Autodesk Inventor part; units mm, degrees
ref_plane "YZ Plane" through (0, 0, 0) normal (1, 0, 0) x (0, 1, 0)
ref_plane "XZ Plane" through (0, 0, 0) normal (0, 1, 0) x (-1, 0, 0)
ref_plane "XY Plane" through (0, 0, 0) normal (0, 0, 1) x (1, 0, 0)
sketch "Sketch1" plane through (0, 0, 0) normal (0, 0, 1) x (1, 0, 0)
  circle A0 centre (0, 0) radius 2.5
  line L0 (0, 0) -> (-10.5, 0)
  circle A1 centre (-10.5, 0) radius 1.5
  arc A2 (-10.5, 5) -> (-10.5, -5) centre (-10.5, 0) ccw
  line L1 (-10.5, 5) -> (0, 5)
  line L2 (0, 5) -> (0, -5)
  line L3 (0, -5) -> (-10.5, -5)
  line L4 (0, 0) -> (0, -10.5)
  circle A3 centre (0, -10.5) radius 1.5
  arc A4 (-5, -10.5) -> (5, -10.5) centre (0, -10.5) ccw
  line L5 (-5, -10.5) -> (-5, 0)
  line L6 (5, 0) -> (5, -10.5)
  line L7 (0, 0) -> (10.5, 0)
  circle A5 centre (10.5, 0) radius 1.5
  arc A6 (10.5, -5) -> (10.5, 5) centre (10.5, 0) ccw
  line L8 (10.5, -5) -> (0, -5)
  line L9 (0, 5) -> (10.5, 5)
  line L10 (0, 0) -> (0, 10.5)
  circle A7 centre (0, 10.5) radius 1.5
  arc A8 (5, 10.5) -> (-5, 10.5) centre (0, 10.5) ccw
  line L11 (5, 10.5) -> (5, 0)
  line L12 (-5, 0) -> (-5, 10.5)
  circle A9 centre (0, 0) radius 4.5
  point P0 (-5, -5)
  point P1 (5, -5)
  point P2 (5, 5)
  point P3 (-5, 5)
  dimension "d0" = 10.5
  dimension "d1" = 3
  dimension "d2" = 5
  dimension "d3" = 10
  dimension "d6" = 360
  dimension "d8" = 9
extrude "Extrusion1" add sketch "Sketch1" against normal blind 2 contours L7 A9 L2 A0 | A0 L2 A9 L7 | A0 L0 A9 L2 | L2 A9 L0 A0 | A9 L2 L9 L11 L7 | L7 L6 L8 L2 A9 | A9 L0 L12 L1 L2 | L2 L3 L5 L0 A9 | L11 L9 A6 L8 L6 | L1 L12 A8 L11 L9 | L8 L6 A4 L5 L3 | L5 L3 A2 L1 L12
extrude "Extrusion2" add sketch "Sketch1" along normal blind 10 contours L7 A9 L2 A0 | A0 L2 A9 L7 | A0 L0 A9 L2 | L2 A9 L0 A0
fillet "Fillet1" radius 1 12 edges at (-7.75, -5, 0) (-7.75, 5, 0) (-15.5, 0, 0) (5, -7.75, 0) (-5, -7.75, 0) (0, -15.5, 0) (15.5, 0, 0) (7.75, 5, 0) (7.75, -5, 0) (-5, 7.75, 0) (5, 7.75, 0) (0, 15.5, 0)
chamfer "Chamfer1" distance 1 angle 45 1 edges at (-4.5, 0, 0)
fillet "Fillet2" radius 1 1 edges at (-4.5, 0, 10)
properties part number "dudukan gps"
Input: part model. Units: mm. Frame: model coordinates. A direction names the side the tool comes from. Coordinates: 2 decimals unless noted, no trailing zeros. Order: outer loops, then holes, each group sorted by start corner. A loop starts at its lowest first (then second) coordinate and runs counter-clockwise, first axis right, second up. Notation, with made-up numbers: (39.25, 59.25) - (45.25, 59.25) arc R28 cw to (45.25, 97.25) - close; hole circle Ø7 at (88.5, 10.25). An arc over 180 degrees is marked (long way). Put each result on its own line as item: value.
1. Reachability of faces 1 (the face through (7.296, -4.699, -0.285)), 2 (the face through (-4.715, -7.204, -0.301)), 3 (the face through (4.715, 7.204, -0.301)), 4 (the face through (7.8, -5, -1.5)), 5 (the face through (-7.204, 4.715, -0.301)) from +Z, -Z, +X, -X, +Y, -Y: full face, straight path, thin tool, end or side. Return the list, or none.
Report:
face 1: +Z, +X, -Y
face 2: +Z, -X, -Y
face 3: +Z, +X, +Y
face 4: +Z, -Z, +X, -Y
face 5: +Z, -X, +Y
2. Line query: line 1 along Y through (x, z) = (0, -1.1); line 2 along X through (y, z) = (-10.5, -1.5); line 3 along X through (y, z) = (0, 1.25). Output: solid intervals per line, ascending.
Report:
line 1: y = -15.5 to -12, -9 to -2.5, 2.5 to 9, 12 to 15.5
line 2: x = -5 to -1.5, 1.5 to 5
line 3: x = -4.5 to -2.5, 2.5 to 4.5
3. Draft query along X for faces 6 (the face through (0, -12, -1)), 7 (the face through (7.7, 5, -1.5)), 8 (the face through (-15.5, 0.1, -1.5)), 9 (the face through (-12, 0, -1)). Return one class per face: pulls with the +X half, pulls with the -X half, needs draft (parallel to the pull), parting line crosses it, or undercut.
Report:
face 6: undercut
face 7: needs draft
face 8: pulls with the -X half
face 9: undercut
4. Cut plane A-A on y = 0. Return the cut outline in (x, z).
Report:
outline: (-15.5, -2) - (-12, -2) - (-12, 0) - (-14.5, 0) arc R1 ccw to (-15.5, -1) - close; (-9, -2) - (-2.5, -2) - (-2.5, 10) - (-3.5, 10) arc R1 ccw to (-4.5, 9) - (-4.5, 1) - (-5.5, 0) - (-9, 0) - close; (2.5, -2) - (9, -2) - (9, 0) - (5.5, 0) - (4.5, 1) - (4.5, 9) arc R1 ccw to (3.5, 10) - (2.5, 10) - close; (12, -2) - (15.5, -2) - (15.5, -1) arc R1 ccw to (14.5, 0) - (12, 0) - close
5. Contact query for flat-ended pins moving along their axis: pin 1 Ø2.5 at (x, y) = (-10.5, 0) entering from -Z; pin 2 Ø0.8 at (x, z) = (-8.5, -1.5) entering from +Y; pin 3 Ø0.5 at (y, z) = (7, -1.5) entering from -X; pin 4 Ø0.8 at (y, z) = (7.5, -1.5) entering from +X. Output: stop coordinate, or through.
Report:
pin 1: passes through
pin 2: stops at y = 5
pin 3: stops at x = -5
pin 4: stops at x = 5
6. Cut plane C-C on z = 5. Return the cut outline in (x, y).
Report:
outline: circle Ø9 at (0, 0); hole circle Ø5 at (0, 0)
7. Cut plane D-D on x = -6. Return the cut outline in (y, z), then the cut area to 3 significant figures.
Report:
outline: (-5, -2) - (5, -2) - (5, -1) arc R1 ccw to (4, 0) - (-4, 0) arc R1 ccw to (-5, -1) - close
area: 19.6 mm2
